```python
from build123d import *

# Parameters (mm, degrees)
IZIM1_R                     = 1.6
IZIM1_R_2                   = 4
IZIM1_R_3                   = 5
Y_KSEKLIK_EKSTR_ZYON1_DEPTH = 3
IZIM2_R                     = 12.1
IZIM2_R_2                   = 11.1
Y_KSEKLIK_EKSTR_ZYON2_DEPTH = 7
IZIM3_R                     = 1.6
KES_EKSTR_ZYON1_DEPTH       = 82.48402276


with BuildPart() as part:
    # Çizim1 → Yükseklik-Ekstrüzyon1 (new body)
    with BuildSketch(Plane(origin=(0, 0, 0), x_dir=(1, 0, 0), z_dir=(0, 1, 0))):
        with BuildLine():
            Line((50.760204115, 37.614624087), (68.08430001, 1.70394254))
            Line((68.08430001, 1.70394254), (68.084798737, -23.286510722))
            ThreePointArc((68.084798737, -23.286510722), (66.158877099, -27.229964111), (61.864685641, -28.135457628))
            Line((61.864685641, -28.135457628), (14.999890892, -16.342900955))
            ThreePointArc((14.999890892, -16.342900955), (8.811960476, -12.013704596), (6.435524315, -4.845373191))
            Line((6.435524315, -4.845373191), (6.435446445, 1.690953534))
            Line((6.435446445, 1.690953534), (6.435084331, 32.216193937))
            ThreePointArc((6.435084331, 32.216193937), (9.949698543, 40.701509037), (18.434929969, 44.216325258))
            Line((18.434929969, 44.216325258), (40.042732612, 44.21658225))
            ThreePointArc((40.042732612, 44.21658225), (46.336600804, 42.433676297), (50.760204115, 37.614624087))
        make_face()
        with Locations(Location((42.260458863, 0.041620293, 0), (0, 0, 90))):
            Circle(IZIM1_R, mode=Mode.SUBTRACT)
        with Locations(Location((19.13547597, 30.841945567, 0), (0, 0, 90))):
            Circle(IZIM1_R_2, mode=Mode.SUBTRACT)
        with Locations(Location((36.135474475, 30.846047168, 0), (0, 0, 90))):
            Circle(IZIM1_R_3, mode=Mode.SUBTRACT)
    extrude(amount=Y_KSEKLIK_EKSTR_ZYON1_DEPTH)

    # Çizim2 → Yükseklik-Ekstrüzyon2 (add)
    with BuildSketch(Plane(origin=(0, 3, 0), x_dir=(1, 0, 0), z_dir=(0, 1, 0))):
        with Locations(Location((36.135474475, 30.846047168, 0), (0, 0, 90))):
            Circle(IZIM2_R)
        with Locations(Location((36.135474475, 30.846047168, 0), (0, 0, 270))):
            Circle(IZIM2_R_2, mode=Mode.SUBTRACT)
    extrude(amount=Y_KSEKLIK_EKSTR_ZYON2_DEPTH)

    # Çizim3 → Kes-Ekstrüzyon1 (cut, through all)
    with BuildSketch(Plane(origin=(0, 3, 0), x_dir=(1, 0, 0), z_dir=(0, 1, 0))):
        with Locations(Location((22.23883129, 40.216370499, 0), (0, 0, 270))):
            Circle(IZIM3_R)
    extrude(amount=-KES_EKSTR_ZYON1_DEPTH, mode=Mode.SUBTRACT)


solid = part.part
```
Work out the finished part from the listing and answer in its coordinate system (mm). A direction names the side the tool comes from. Give positions to 0.01 mm unless a question says otherwise; leave off trailing zeros. Write each loop counter-clockwise with the first axis right and the second up, starting at its lowest first coordinate (ties: lowest second). Pieces come first, ordered by that corner, then holes.
(1) Straight lines are drawn through the part: line 1 (Y direction, x = 47, z = -1.5); line 2 (X direction, y = 7, z = -36); line 3 (X direction, y = 3.5, z = -33). For each, find the intervals that lie inside material, in ascending order.
Final values:
line 1: y = 0 to 3
line 2: x = 25.19 to 26.3, 45.97 to 47.08
line 3: x = 24.23 to 25.25, 47.02 to 48.04
(2) The part is cut by section D-D on x = 28.5. Write down the section's boundary in (y, z).
Final values:
outline: (0, -44.22) - (3, -44.22) - (3, -40.23) - (10, -40.23) - (10, -38.9) - (3, -38.9) - (3, -22.79) - (10, -22.79) - (10, -21.46) - (3, -21.46) - (3, 19.74) - (0, 19.74) - close
(3) The part is cut by section C-C on y = 6. Write down the section's boundary in (x, z), plus the area to 3 significant figures.
Final values:
outline: circle Ø24.2 at (36.14, -30.85); hole circle Ø22.2 at (36.14, -30.85)
area: 72.9 mm2
(4) The part is cut by section B-B on z = -34. Write down the section's boundary in (x, y), plus the area to 3 significant figures.
Final values:
outline: (6.57, 0) - (16.68, 0) - (16.68, 3) - (6.57, 3) - close; (21.59, 0) - (32.26, 0) - (32.26, 3) - (25.49, 3) - (25.49, 10) - (24.45, 10) - (24.45, 3) - (21.59, 3) - close; (40.02, 0) - (52.5, 0) - (52.5, 3) - (47.82, 3) - (47.82, 10) - (46.78, 10) - (46.78, 3) - (40.02, 3) - close
area: 114 mm2
(5) Which of the six approach directions +Z, -Z, +X, -X, +Y, -Y give full straight-line access (tool end or side, diameter ignored) to faces 1 (the cylindrical face through (36.624, 6.451, -41.935)), 2 (the cylindrical face through (31.178, 1.479, -30.195))?
Final values:
face 1: +Y
face 2: +Y, -Y
(6) The part is cut by section A-A on x = 37. Write down the section's boundary in (y, z).
Final values:
outline: (0, -44.22) - (3, -44.22) - (3, -42.92) - (10, -42.92) - (10, -41.91) - (3, -41.91) - (3, -35.77) - (0, -35.77) - close; (0, -25.92) - (3, -25.92) - (3, -19.78) - (10, -19.78) - (10, -18.78) - (3, -18.78) - (3, 21.88) - (0, 21.88) - close
(7) The mould has two halves that part along X. Classify faces 3 (the flat face through (38, 3, -8)), 4 (the cylindrical face through (27.958, 6.451, -21.928)), 5 (the cylindrical face through (18.96, 1.479, -26.846)): pulls with the +X half, pulls with the -X half, needs draft (parallel to the pull), parting line crosses it, or undercut.
Final values:
face 3: needs draft
face 4: parting line crosses it
face 5: undercut
(8) Flat-ended cylindrical pins translate along their axes: pin 1 Ø4 at (x, y) = (37, 6) entering from +Z; pin 2 Ø5 at (x, z) = (51.5, -17.5) entering from -Y; pin 3 Ø5 at (x, z) = (55, -11) entering from +Y; pin 4 Ø7 at (x, z) = (19.14, -30.84) entering from -Y. Find the tip coordinate at first contact, or state that the pin passes through.
Final values:
pin 1: stops at z = -18.75
pin 2: stops at y = 0
pin 3: stops at y = 3
pin 4: passes through
